Autodesk Inventor part; units mm, degrees
ref_plane "YZ Plane" through (0, 0, 0) normal (1, 0, 0) x (0, 1, 0)
ref_plane "XZ Plane" through (0, 0, 0) normal (0, 1, 0) x (-1, 0, 0)
ref_plane "XY Plane" through (0, 0, 0) normal (0, 0, 1) x (1, 0, 0)
sketch "Boceto1" plane through (0, 0, 0) normal (0, 1, 0) x (-1, 0, 0)
  arc A0 (119.9994, -35.5039) -> (120.0001, -24.5039) centre (119.9998, -30.0039) ccw
  arc A1 (62, -24.5) -> (61.9993, -35.5) centre (61.9996, -30) ccw
  line L0 (62, -24.5) -> (120.0001, -24.5039)
  line L1 (119.9994, -35.5039) -> (61.9993, -35.5)
  circle A2 centre (119.9998, -30.0039) radius 1.5
  circle A3 centre (61.9996, -30) radius 1.5
  point P0 (124.9998, -30.0039)
  point P1 (119.9998, -25.0039)
  dimension "d172" = 3
  dimension "d173" = 3
extrude "Extrusión1" add sketch "Boceto1" along normal blind 3
properties part number "biela"
For this review, take the finished solid that the model builds, in its own axes (mm). Coordinates: 2 decimals unless noted, no trailing zeros. Loops run counter-clockwise (first coordinate to the right, second up) from the corner with the lowest first, then second, coordinate; pieces in that order, holes last. Notation, with made-up numbers: (34, 30) - (40, 30) arc R25 cw to (40, 47) - close; hole circle Ø5 at (14, 21). An arc over 180 degrees is marked (long way). Use one line per item in the form item = value. Start each with the question number.
1) Take a section at C-C (z = -33.25). State the section outline as (x, y) points, plus the area to 3 significant figures.
2) Draft analysis for pull direction Z (two halves, no side actions). For faces 1 (the face through (-91, 3, -30)), 2 (the face through (-56.5, 1.5, -30.1)), 3 (the face through (-121.43, 1.48, -30.45)), state which applies: released by +Z, released by -Z, zero draft, split by the parting line, or undercut.
3) To check wall thickness, follow probe 1 along Z at (x, y) = (-74, 2.75); probe 2 along X at (y, z) = (0.85, -30.25); probe 3 along X at (y, z) = (2.6, -30.5). State the ranges of each line that lie inside material, in increasing order. Write a range as from..to.
4) Take a section at B-B (z = -25.5). State the section outline as (x, y) points.
5) For pin 1 (4 mm diameter, centred on x = -120, z = -30, fed in from +Y), flat-tipped, find the tip position at first contact; note if it passes through.
6) Take a section at A-A (y = 1.5). State the section outline as (x, z) points, plus the area to 3 significant figures.
From the geometry:
q1.outline = (-124.44, 0) - (-57.56, 0) - (-57.56, 3) - (-124.44, 3) - close
q1.area = 201 mm2
q2.face_1 = zero draft
q2.face_2 = split by the parting line
q2.face_3 = undercut
q3.probe_1 = -35.5..-24.5
q3.probe_2 = -125.49..-121.48, -118.52..-63.48, -60.52..-56.51
q3.probe_3 = -125.48..-121.42, -118.58..-63.41, -60.59..-56.52
q4.outline = (-123.16, 0) - (-58.84, 0) - (-58.84, 3) - (-123.16, 3) - close
q5.pin_1 = 3
q6.outline = (-120, -35.5) - (-62, -35.5) arc R5.5 ccw to (-62, -24.5) - (-120, -24.5) arc R5.5 ccw to start; hole circle Ø3 at (-120, -30); hole circle Ø3 at (-62, -30)
q6.area = 719 mm2
